from build123d import *

# Parameters (mm, degrees)
F1_DEPTH  = 102.5
F2_R      = 3.5
F3_DEPTH  = 2
F5_DEPTH  = 5
F6_R      = 1
F8_DEPTH  = 16
F10_DEPTH = 2


with BuildPart() as f1:
    # F0 (on Front) → F1 (new body, symmetric)
    with BuildSketch(Plane.XZ):
        Polygon((55, 70), (0, 70), (-55, 70), (-70, 65), (-70, 0), (-68, 0), (0, 0), (68, 0), (70, 0), (70, 65), align=None)
        with BuildLine():
            Line((70, -3), (70, 0))
            Line((70, 0), (68, 0))
            Line((68, 0), (68, -5))
            ThreePointArc((68, -5), (68.87868, -7.12132), (71, -8))
            Line((71, -8), (82, -8))
            Line((82, -8), (82, -6))
            Line((82, -6), (73, -6))
            ThreePointArc((73, -6), (70.87868, -5.12132), (70, -3))
        make_face()
        with BuildLine():
            Line((-68, 0), (-70, 0))
            Line((-70, 0), (-70, -3))
            ThreePointArc((-70, -3), (-70.87868, -5.12132), (-73, -6))
            Line((-73, -6), (-82, -6))
            Line((-82, -6), (-82, -8))
            Line((-82, -8), (-71, -8))
            ThreePointArc((-71, -8), (-68.87868, -7.12132), (-68, -5))
            Line((-68, -5), (-68, 0))
        make_face()
    extrude(amount=F1_DEPTH, both=True)

    # F2 (on face) → F3 (cut, through all)
    with BuildSketch(Plane.XY.offset(-6)):
        with Locations((77.5, -97)):
            Circle(F2_R)
        with Locations((77.5, 97)):
            Circle(F2_R)
        with Locations((-77.5, -97)):
            Circle(F2_R)
        with Locations((-77.5, 97)):
            Circle(F2_R)
    extrude(amount=-F3_DEPTH, mode=Mode.SUBTRACT)

    # F4 (on face) → F5 (join)
    with BuildSketch(Plane.XZ.offset(102.5)):
        with BuildLine():
            Line((50, 57), (23, 57))
            ThreePointArc((23, 57), (20.87868, 56.12132), (20, 54))
            Line((20, 54), (20, 38))
            ThreePointArc((20, 38), (20.87868, 35.87868), (23, 35))
            Line((23, 35), (50, 35))
            ThreePointArc((50, 35), (52.12132, 35.87868), (53, 38))
            Line((53, 38), (53, 54))
            ThreePointArc((53, 54), (52.12132, 56.12132), (50, 57))
        make_face()
    extrude(amount=F5_DEPTH)

    # F6
    f6_edges = [f1.edges().sort_by_distance(p)[0] for p in [
        (36.5, -107.5, 57),
        (20.87868, -107.5, 56.12132),
        (20, -107.5, 46),
        (20.87868, -107.5, 35.87868),
        (36.5, -107.5, 35),
        (52.12132, -107.5, 35.87868),
        (53, -107.5, 46),
        (52.12132, -107.5, 56.12132),
    ]]
    fillet(f6_edges, radius=F6_R)

    # F7 (on face) → F8 (cut)
    with BuildSketch(Plane.XZ.offset(107.5)):
        Polygon((43, 53), (30, 53), (24, 48), (24, 39), (49, 39), (49, 48), align=None)
    extrude(amount=-F8_DEPTH, mode=Mode.SUBTRACT)

    # F9 (on face) → F10 (cut)
    with BuildSketch(Plane.XZ.offset(102.5)):
        with BuildLine():
            Line((17, 22.5), (17, 47.5))
            ThreePointArc((17, 47.5), (9.98097, 57.98097), (-0.5, 65))
            Line((-0.5, 65), (-25.5, 65))
            ThreePointArc((-25.5, 65), (-35.98097, 57.98097), (-43, 47.5))
            Line((-43, 47.5), (-43, 22.5))
            ThreePointArc((-43, 22.5), (-35.98097, 12.01903), (-25.5, 5))
            Line((-25.5, 5), (-0.5, 5))
            ThreePointArc((-0.5, 5), (9.98097, 12.01903), (17, 22.5))
        make_face()
    extrude(amount=-F10_DEPTH, mode=Mode.SUBTRACT)


solid = f1.part
CAD build for the part. Positions are in the model's coordinates, mm. A direction names the side the tool comes from. Give positions to 0.01 mm unless a question says otherwise; leave off trailing zeros. Write each loop counter-clockwise with the first axis right and the second up, starting at its lowest first coordinate (ties: lowest second). Pieces come first, ordered by that corner, then holes. Notation, with made-up numbers: (-1.75, -20.5) -> (6.25, -20.5) arc R14 ccw to (6.25, 6.5) -> close; hole circle Ø1 at (34.5, -25.5). An arc over 180 degrees is marked (long way). Return JSON: item names as keys, results as strings.
Item 1: Band-saw the part on B-B (x = 77.5). List the corners of the cut face in (y, z).
Answer below:
{"outline": "(-102.5, -8) -> (-100.5, -8) -> (-100.5, -6) -> (-102.5, -6) -> close; (-93.5, -8) -> (93.5, -8) -> (93.5, -6) -> (-93.5, -6) -> close; (100.5, -8) -> (102.5, -8) -> (102.5, -6) -> (100.5, -6) -> close"}
Item 2: Drill centre lines: probe 1 along Y at (x, z) = (77.5, -7); probe 2 along X at (y, z) = (-50, -1); probe 3 along Z at (x, y) = (12.5, -90.5). Where is each one in solid material? Low to high.
Answer below:
{"probe 1": "y = -102.5 to -100.5, -93.5 to 93.5, 100.5 to 102.5", "probe 2": "x = -70 to -68, 68 to 70", "probe 3": "z = 0 to 70"}
Item 3: Band-saw the part on D-D (z = 32.5). List the corners of the cut face in (x, y).
Answer below:
{"outline": "(-70, -102.5) -> (-43, -102.5) -> (-43, -100.5) -> (17, -100.5) -> (17, -102.5) -> (70, -102.5) -> (70, 102.5) -> (-70, 102.5) -> close"}
Item 4: Band-saw the part on A-A (y = -97). Give the number of separate pieces and of enclosed holes in the cut face, then the cut area to 3 significant figures.
Answer below:
{"separate pieces": "3", "enclosed holes": "1", "area": "9,460 mm2"}
Item 5: Drop flat-ended pins along their axis: pin 1 (1.6 mm diameter, centred on y = -101, z = 33, fed in from +X); pin 2 (2 mm diameter, centred on x = -19, z = 59.5, fed in from -Y); pin 3 (1.2 mm diameter, centred on x = 30, y = -105, fed in from +Z). Give the stop position or say it passes through.
Answer below:
{"pin 1": "stops at x = 70", "pin 2": "stops at y = -100.5", "pin 3": "stops at z = 57"}
Item 6: Two-plate mould, pull along Z, no slides. Class faces 6 (the flat face through (37, -100, 53)), 7 (the flat face through (78, -1, -6)), 8 (the cylindrical face through (-75.885, -100.105, -6.986)): +Z half, -Z half, draft (parallel to the pull), parting line (faces both ways), or undercut.
Answer below:
{"face 6": "undercut", "face 7": "+Z half", "face 8": "draft"}
Item 7: Tool access for faces 1 (the flat face through (70, -1, 31)), 2 (the flat face through (-70, -1, 31)), 3 (the flat face through (-1, 102.5, 32)), 4 (the flat face through (-13, -100.5, 35)), 5 (the flat face through (-68, -1, -3)): list every direction of +Z, -Z, +X, -X, +Y, -Y with a clear straight run to the whole face (end or side of a thin tool).
Answer below:
{"face 1": "+Z, +X, +Y, -Y", "face 2": "+Z, -X, +Y, -Y", "face 3": "+Z, -Z, +X, -X, +Y", "face 4": "-Y", "face 5": "-Z, +Y, -Y"}
Item 8: Band-saw the part on C-C (x = -39). List the corners of the cut face in (y, z), then the cut area to 3 significant figures.
Answer below:
{"outline": "(-102.5, 0) -> (102.5, 0) -> (102.5, 70) -> (-102.5, 70) -> (-102.5, 54.5) -> (-100.5, 54.5) -> (-100.5, 15.5) -> (-102.5, 15.5) -> close", "area": "14,300 mm2"}
